Source: three-view drawing plus pictorial views. Frame: mm from the lowest corner of the part. A direction names the side the tool comes from. Round coordinates to 2 decimals unless told otherwise and drop trailing zeros. Loops run counter-clockwise (first coordinate to the right, second up) from the corner with the lowest first, then second, coordinate; pieces in that order, holes last. Notation, with made-up numbers: (68.25, 39) -> (76.25, 39) arc R22 cw to (76.25, 74) -> close; hole circle Ø8 at (15, 1.25). An arc over 180 degrees is marked (long way). Put each result on its own line as item: value. Start each with the question number.
1. Cut plane C-C (x = 18.25). Return the cut outline in (y, z), then the cut area to 3 significant figures.
2. Material intervals for L1, parallel to X at y = 7.75, z = 8.25; L2, parallel to X at y = 5.5, z = 3.5; L3, parallel to Z at x = 23, y = 9.25, sorted ascending.
3. Cut plane A-A (y = 4.25). Return the cut outline in (x, z), then the cut area to 3 significant figures.
4. Draft query along X for the marked faces 1, 2 and 3. Return one class per face: pulls with the +X half, pulls with the -X half, needs draft (parallel to the pull), parting line crosses it, or undercut.
5. Cut plane B-B (z = 3). Return the cut outline in (x, y), then the cut area to 3 significant figures.
6. Cut plane D-D (z = 7.75). Return the cut outline in (x, y).
7. Set-up query: the marked faces 4, 5 and 6. Return all of +Z, -Z, +X, -X, +Y, -Y with unobstructed straight access to the full face (end or side cutting, diameter ignored); none if empty.
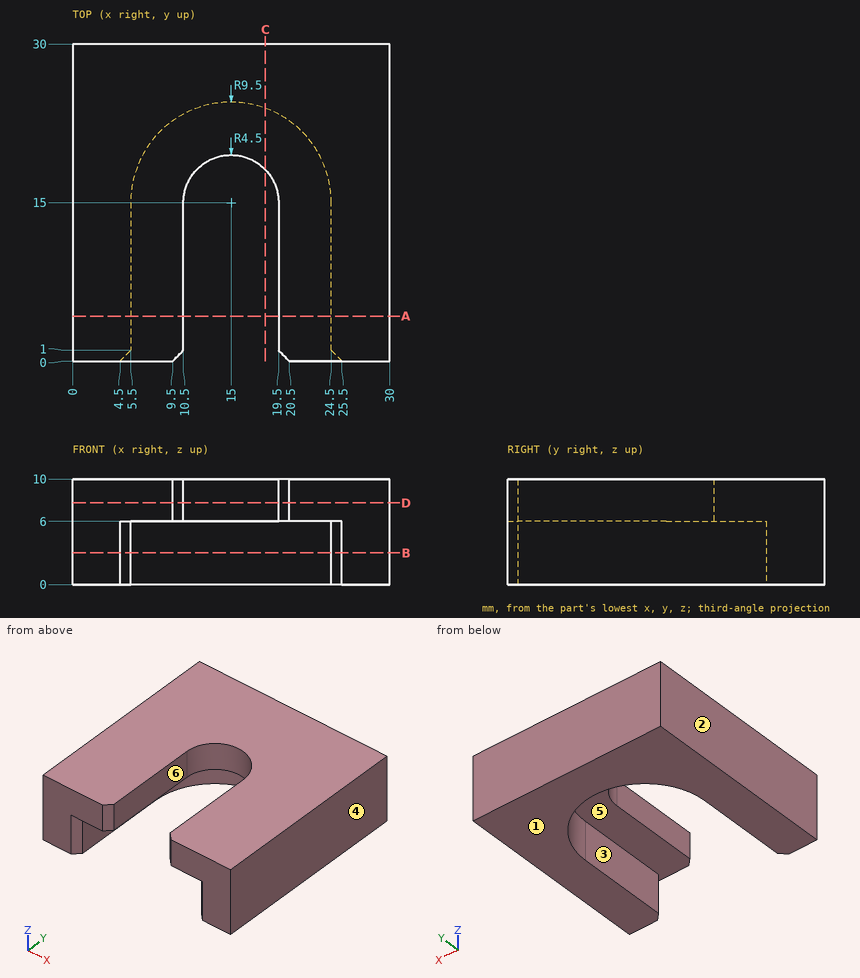
Solution:
1. outline: (18.11, 6) -> (23.93, 6) -> (23.93, 0) -> (30, 0) -> (30, 10) -> (18.11, 10) -> close
1. area: 84.0 mm^2
2. L1: x = 0 to 10.5, 19.5 to 30
2. L2: x = 0 to 5.5, 24.5 to 30
2. L3: z = 6 to 10
3. outline: (0, 0) -> (5.5, 0) -> (5.5, 6) -> (10.5, 6) -> (10.5, 10) -> (0, 10) -> close; (19.5, 6) -> (24.5, 6) -> (24.5, 0) -> (30, 0) -> (30, 10) -> (19.5, 10) -> close
3. area: 150 mm^2
4. face 1: needs draft
4. face 2: pulls with the -X half
4. face 3: undercut
5. outline: (0, 0) -> (4.5, 0) -> (5.5, 1) -> (5.5, 15) arc R9.5 cw to (24.5, 15) -> (24.5, 1) -> (25.5, 0) -> (30, 0) -> (30, 30) -> (0, 30) -> close
5. area: 472 mm^2
6. outline: (0, 0) -> (9.5, 0) -> (10.5, 1) -> (10.5, 15) arc R4.5 cw to (19.5, 15) -> (19.5, 1) -> (20.5, 0) -> (30, 0) -> (30, 30) -> (0, 30) -> close
7. face 4: +Z, -Z, +X, +Y, -Y
7. face 5: -Z, -Y
7. face 6: +Z, -Z, -Y
